Check sheet for the modelled part. Datum: model origin and axes. Units: mm. Round coordinates to 2 decimals unless told otherwise and drop trailing zeros. Loops run counter-clockwise (first coordinate to the right, second up) from the corner with the lowest first, then second, coordinate; pieces in that order, holes last. Notation, with made-up numbers: M 84.25,33 L 130.25,33 A25 ccw 130.25,47 Z; hole C -30.5,87 d8. An arc over 180 degrees is marked long. One line per question, with ' | ' between items. Start each with the question number.
(1) Section check B-B (x = -190.5). Record the boundary of the cut face in (y, z) (3 decimals), and give its area (3 significant figures).
(2) Thickness scan on probe 1 along Z at (x, y) = (-190.5, 3.05) (3 decimals); probe 2 along Z at (x, y) = (-192.5, 3); probe 3 along X at (y, z) = (2.45, -304.8) (3 decimals). Record the ranges inside material, lowest first. Write a range as [from, to].
(3) Section check D-D (x = -83.82). Record the boundary of the cut face in (y, z) (3 decimals).
(4) Section check A-A (y = 2.45). Record the boundary of the cut face in (x, z) (3 decimals), and give its area (3 significant figures).
(5) Section check C-C (z = -368.3). Record the boundary of the cut face in (x, y) (3 decimals), and give its area (3 significant figures).
(6) Go/stop test with a flat-tipped pin: P1, Ø7.5, axis at x = -116.84, z = -368.3, coming from the +Y side. Record where the tip stops, or that it passes through.
(7) Draft check along X on faces 1 (the face through (-189.55, 2.58, -365.27)), 2 (the face through (-94.6, 2.5, -329)), 3 (the face through (-155, 3, -381)). Enter one of: +X half, -X half, draft (parallel to the pull), parting line (faces both ways), or undercut.
```python
from build123d import *

# Parameters (mm, degrees)
BOSS_EXTRUDE1_DEPTH = 5.08
SKETCH2_R           = 3.175
CUT_EXTRUDE1_DEPTH  = 5.08


with BuildPart() as part:
    # Sketch1 → Boss-Extrude1 (new body)
    with BuildSketch(Plane(origin=(0, 0, 0), x_dir=(1, 0, 0), z_dir=(0, 1, 0))):
        with BuildLine():
            Line((-203.2, 381), (-203.2, 177.143917216))
            ThreePointArc((-203.2, 177.143917216), (-151.025197649, 259.077837422), (-59.18865855, 290.723174629))
            ThreePointArc((-59.18865855, 290.723174629), (-94.980572199, 329.698017536), (-107.95, 381))
            Line((-107.95, 381), (-203.2, 381))
        make_face()
    extrude(amount=BOSS_EXTRUDE1_DEPTH)

    # Sketch2 → Cut-Extrude1 (cut)
    with BuildSketch(Plane(origin=(0, 5.08, 0), x_dir=(1, 0, 0), z_dir=(0, 1, 0))):
        with Locations(Location((-190.5, 233.68, 0), (0, 0, 270))):
            Circle(SKETCH2_R)
        with Locations(Location((-83.82, 302.26, 0), (0, 0, 270))):
            Circle(SKETCH2_R)
        with Locations(Location((-116.84, 368.3, 0), (0, 0, 270))):
            Circle(SKETCH2_R)
        with Locations(Location((-190.5, 368.3, 0), (0, 0, 270))):
            Circle(SKETCH2_R)
        with Locations(Location((-142.24, 281.94, 0), (0, 0, 270))):
            Circle(SKETCH2_R)
        with Locations(Location((-190.5, 304.8, 0), (0, 0, 270))):
            Circle(SKETCH2_R)
    extrude(amount=-CUT_EXTRUDE1_DEPTH, mode=Mode.SUBTRACT)


solid = part.part
```
The answers:
1) outline: M 0,-381 L 5.08,-381 L 5.08,-371.475 L 0,-371.475 Z; M 0,-365.125 L 5.08,-365.125 L 5.08,-307.975 L 0,-307.975 Z; M 0,-301.625 L 5.08,-301.625 L 5.08,-236.855 L 0,-236.855 Z; M 0,-230.505 L 5.08,-230.505 L 5.08,-211.372 L 0,-211.372 Z | area: 765 mm²
2) probe 1: [-381, -371.475], [-365.125, -307.975], [-301.625, -236.855], [-230.505, -211.372] | probe 2: [-381, -370.77], [-365.83, -307.27], [-302.33, -236.15], [-231.21, -207.38] | probe 3: [-203.2, -193.675], [-187.325, -85.725], [-81.915, -76.464]
3) outline: M 0,-312.975 L 5.08,-312.975 L 5.08,-305.435 L 0,-305.435 Z; M 0,-299.085 L 5.08,-299.085 L 5.08,-288.752 L 0,-288.752 Z
4) outline: M -203.2,-381 L -107.95,-381 A107.95 cw -59.189,-290.723 A147.32 cw -203.2,-177.144 Z; hole C -190.5,-368.3 d6.35; hole C -190.5,-304.8 d6.35; hole C -190.5,-233.68 d6.35; hole C -142.24,-281.94 d6.35; hole C -116.84,-368.3 d6.35; hole C -83.82,-302.26 d6.35 | area: 13,900 mm²
5) outline: M -203.2,0 L -193.675,0 L -193.675,5.08 L -203.2,5.08 Z; M -187.325,0 L -120.015,0 L -120.015,5.08 L -187.325,5.08 Z; M -113.665,0 L -107.2,0 L -107.2,5.08 L -113.665,5.08 Z | area: 423 mm²
6) P1: y = 5.08
7) face 1: undercut | face 2: +X half | face 3: draft
